For this review, take the finished solid that the model builds, in its own axes (mm). A direction names the side the tool comes from. Give positions to 0.01 mm unless a question says otherwise; leave off trailing zeros. Loops run counter-clockwise (first coordinate to the right, second up) from the corner with the lowest first, then second, coordinate; pieces in that order, holes last. Notation, with made-up numbers: (40.25, 69.25) - (44.25, 69.25) arc R34 cw to (44.25, 106.25) - close; hole circle Ø2 at (42, -6.75). An arc over 180 degrees is marked (long way). Put each result on its own line as item: value.
from build123d import *

# Parameters (mm, degrees)
SKETCH1_W           = 10
SKETCH1_H           = 141
BOSS_EXTRUDE1_DEPTH = 8
SKETCH2_R           = 2.5
CUT_EXTRUDE1_DEPTH  = 8
SKETCH3_W           = 142
SKETCH3_H           = 141
BOSS_EXTRUDE2_DEPTH = 1.5
CUT_EXTRUDE4_DEPTH  = 24
SKETCH12_W          = 60
SKETCH12_H          = 10.777657791
SKETCH12_H_2        = 10.436358021
CUT_EXTRUDE6_DEPTH  = 10
SKETCH14_W          = 22
SKETCH14_H          = 20
BOSS_EXTRUDE5_DEPTH = 6.5
SKETCH16_W          = 61.380351881
SKETCH16_H          = 10.777657791
SKETCH16_H_2        = 10.440898972
CUT_EXTRUDE9_DEPTH  = 26.5
SKETCH17_R          = 4.5
CUT_EXTRUDE10_DEPTH = 3
SKETCH9_R           = 1.25
CUT_EXTRUDE11_DEPTH = 14
SKETCH13_R          = 2.5
CUT_EXTRUDE12_DEPTH = 14
SKETCH19_R          = 4.5
CUT_EXTRUDE13_DEPTH = 4
SKETCH20_R          = 1.25
CUT_EXTRUDE14_DEPTH = 4


with BuildPart() as part:
    # Sketch1 → Boss-Extrude1 (new body)
    with BuildSketch(Plane.XY):
        with Locations((5, 70.5)):
            Rectangle(SKETCH1_W, SKETCH1_H)
    extrude(amount=BOSS_EXTRUDE1_DEPTH)

    # Sketch2 → Cut-Extrude1 (cut)
    with BuildSketch(Plane.XY.offset(8)):
        with Locations((5, 131)):
            Circle(SKETCH2_R)
        with Locations((5, 10)):
            Circle(SKETCH2_R)
    extrude(amount=-CUT_EXTRUDE1_DEPTH, mode=Mode.SUBTRACT)

    # Sketch3 → Boss-Extrude2 (add)
    with BuildSketch(Plane.XY.offset(8)):
        with Locations((81, 70.5)):
            Rectangle(SKETCH3_W, SKETCH3_H)
    extrude(amount=-BOSS_EXTRUDE2_DEPTH)

    # Sketch8 → Cut-Extrude4 (cut)
    with BuildSketch(Plane.XY.offset(8)):
        with BuildLine():
            Line((19.143151415, 136), (125, 136))
            ThreePointArc((125, 136), (130, 131), (125, 126))
            Line((125, 126), (19.143151415, 126))
            ThreePointArc((19.143151415, 126), (14.143151415, 131), (19.143151415, 136))
        make_face()
        with BuildLine():
            Line((19.143151415, 14.495923054), (125, 14.495923054))
            ThreePointArc((125, 14.495923054), (130, 9.495923054), (125, 4.495923054))
            Line((125, 4.495923054), (19.143151415, 4.495923054))
            ThreePointArc((19.143151415, 4.495923054), (14.143151415, 9.495923054), (19.143151415, 14.495923054))
        make_face()
    extrude(amount=-CUT_EXTRUDE4_DEPTH, mode=Mode.SUBTRACT)

    # Sketch12 → Cut-Extrude6 (cut)
    with BuildSketch(Plane.XY.offset(8)):
        with Locations((121.8, 93.584876831)):
            Rectangle(SKETCH12_W, SKETCH12_H)
        with Locations((121.8, 48.647743856)):
            Rectangle(SKETCH12_W, SKETCH12_H_2)
    extrude(amount=-CUT_EXTRUDE6_DEPTH, mode=Mode.SUBTRACT)

    # Sketch14 → Boss-Extrude5 (add)
    with BuildSketch(Plane(origin=(0, 0, 6.5), x_dir=(-1, 0, 0), z_dir=(0, 0, -1))):
        with Locations((-141, 131)):
            Rectangle(SKETCH14_W, SKETCH14_H)
        with Locations((-141, 10)):
            Rectangle(SKETCH14_W, SKETCH14_H)
    extrude(amount=BOSS_EXTRUDE5_DEPTH)

    # Sketch16 → Cut-Extrude9 (cut)
    with BuildSketch(Plane.XY.offset(8)):
        with Locations((122.490175941, 93.584876831)):
            Rectangle(SKETCH16_W, SKETCH16_H)
        with Locations((122.490175941, 48.64547338)):
            Rectangle(SKETCH16_W, SKETCH16_H_2)
    extrude(amount=-CUT_EXTRUDE9_DEPTH, mode=Mode.SUBTRACT)

    # Sketch17 → Cut-Extrude10 (cut)
    with BuildSketch(Plane.XY.offset(8)):
        with Locations((5, 131)):
            Circle(SKETCH17_R)
        with Locations((5, 10)):
            Circle(SKETCH17_R)
    extrude(amount=-CUT_EXTRUDE10_DEPTH, mode=Mode.SUBTRACT)

    # Sketch9 → Cut-Extrude11 (cut)
    with BuildSketch(Plane.XY.offset(8)):
        with Locations((147.028762267, 114.00755189)):
            Circle(SKETCH9_R)
        with Locations((3.027444188, 114)):
            Circle(SKETCH9_R)
        with Locations((3, 30.019439847)):
            Circle(SKETCH9_R)
        with Locations((147, 30.019439847)):
            Circle(SKETCH9_R)
    extrude(amount=-CUT_EXTRUDE11_DEPTH, mode=Mode.SUBTRACT)

    # Sketch13 → Cut-Extrude12 (cut)
    with BuildSketch(Plane.XY.offset(8)):
        with Locations((142, 131)):
            Circle(SKETCH13_R)
        with Locations((142, 10)):
            Circle(SKETCH13_R)
    extrude(amount=-CUT_EXTRUDE12_DEPTH, mode=Mode.SUBTRACT)

    # Sketch19 → Cut-Extrude13 (cut)
    with BuildSketch(Plane.XY.offset(8)):
        with Locations((142, 131)):
            Circle(SKETCH19_R)
        with Locations((142, 10)):
            Circle(SKETCH19_R)
    extrude(amount=-CUT_EXTRUDE13_DEPTH, mode=Mode.SUBTRACT)

    # Sketch20 → Cut-Extrude14 (cut)
    with BuildSketch(Plane.XY.offset(8)):
        with Locations((25, 121)):
            Circle(SKETCH20_R)
        with Locations((130, 121)):
            Circle(SKETCH20_R)
        with Locations((130, 24)):
            Circle(SKETCH20_R)
        with Locations((25, 24)):
            Circle(SKETCH20_R)
    extrude(amount=-CUT_EXTRUDE14_DEPTH, mode=Mode.SUBTRACT)


solid = part.part
1) Take a section at D-D on y = 69. State the section outline as (x, z) points.
Geometry check:
outline: (0, 0) - (10, 0) - (10, 6.5) - (152, 6.5) - (152, 8) - (0, 8) - close
2) Wall thickness on line 1 (Y direction, x = 25, z = 7.1); line 2 (Y direction, x = 56.5, z = 7.75); line 3 (X direction, y = 30, z = 2): over which ranges is each line inside the solid? List them lowest first.
Geometry check:
line 1: y = 0 to 4.5, 14.5 to 22.75, 25.25 to 119.75, 122.25 to 126, 136 to 141
line 2: y = 0 to 4.5, 14.5 to 126, 136 to 141
line 3: x = 0 to 1.75, 4.25 to 10
3) Take a section at C-C on y = 51.5. State the section outline as (x, z) points, and give its area (3 significant figures).
Geometry check:
outline: (0, 0) - (10, 0) - (10, 6.5) - (91.8, 6.5) - (91.8, 8) - (0, 8) - close
area: 203 mm²
4) For faces 1 (the face through (141, 20, 3)), 2 (the face through (130, 9.6, 7.3)), 3 (the face through (146.16, 8.28, 6.03)), 4 (the face through (130, 10, 3)), list the 3-axis set-ups (+Z, -Z, +X, -X, +Y, -Y) from which the entire face can be reached by the end or side of a thin tool; tool diameter is ignored.
Geometry check:
face 1: -Z, +X
face 2: +Z, -Z
face 3: +Z
face 4: -Z, +Y, -Y
5) Insertion check: pin 1 Ø7 at (x, y) = (142, 131) entering from +Z; pin 2 Ø1.5 at (y, z) = (59, 4) entering from -X; pin 3 Ø4.5 at (x, y) = (142, 131) entering from -Z; pin 4 Ø1.2 at (y, z) = (50, 7.5) entering from +X. Each pin has a flat end and moves straight along its axis. Give the tip position at first contact, or say it passes through.
Geometry check:
pin 1: stops at z = 4
pin 2: stops at x = 0
pin 3: passes through
pin 4: stops at x = 91.8
6) Take a section at B-B on x = 41.5. State the section outline as (y, z) points.
Geometry check:
outline: (0, 6.5) - (4.5, 6.5) - (4.5, 8) - (0, 8) - close; (14.5, 6.5) - (126, 6.5) - (126, 8) - (14.5, 8) - close; (136, 6.5) - (141, 6.5) - (141, 8) - (136, 8) - close
7) Take a section at A-A on x = 142. State how many separate pieces and enclosed holes the cut face has, and give its area (3 significant figures).
Geometry check:
separate pieces: 5
enclosed holes: 0
area: 328 mm²
8) Draft analysis for pull direction X (two halves, no side actions). For faces 5 (the face through (14.144, 9.386, 7.26)), 6 (the face through (139, 10, 0)), 7 (the face through (152, 129, 5)), state which applies: pulls with the +X half, pulls with the -X half, needs draft (parallel to the pull), parting line crosses it, or undercut.
Geometry check:
face 5: undercut
face 6: needs draft
face 7: pulls with the +X half
